Input: part model. Units: mm. Frame: model coordinates. A direction names the side the tool comes from. Round coordinates to 2 decimals unless told otherwise and drop trailing zeros. Write each loop counter-clockwise with the first axis right and the second up, starting at its lowest first coordinate (ties: lowest second). Pieces come first, ordered by that corner, then holes. Notation, with made-up numbers: (22, 20.25) - (47, 20.25) arc R25 ccw to (47, 33.25) - close; hole circle Ø8 at (60.25, 83). An arc over 180 degrees is marked (long way). Use one line per item in the form item = value.
```python
from build123d import *

# Parameters (mm, degrees)
SKETCH1_W           = 40
SKETCH1_H           = 40
SKETCH1_R           = 1.5
SKETCH1_R_2         = 2.8
BOSS_EXTRUDE1_DEPTH = 5.7
BOSS_EXTRUDE3_START = 5.7
SKETCH1_3_W         = 40
SKETCH1_3_H         = 40
SKETCH1_3_R         = 2.8
SKETCH1_3_R_2       = 1.5
BOSS_EXTRUDE3_DEPTH = 3.4
SKETCH4_W           = 3.5
SKETCH4_H           = 40
CUT_EXTRUDE2_DEPTH  = 4
SKETCH2_W           = 3
SKETCH2_H           = 40
BOSS_EXTRUDE4_DEPTH = 5.1
CUT_EXTRUDE3_START  = -39.5
SKETCH5_R           = 2
CUT_EXTRUDE3_DEPTH  = 33
CUT_EXTRUDE4_START  = -5.1
SKETCH6_W           = 3.85
SKETCH6_H           = 5.76
CUT_EXTRUDE4_DEPTH  = 5.1
FILLET1_R           = 0.62
CHAMFER1_SIZE       = 1.4
CHAMFER1_SIZE2      = 3.144451483


with BuildPart() as part:
    # Sketch1 → Boss-Extrude1 (new body)
    # profile 1 of 7: a face of its own
    with BuildSketch(Plane(origin=(0, 0, 0), x_dir=(1, 0, 0), z_dir=(0, 1, 0))):
        Rectangle(SKETCH1_W, SKETCH1_H)
        with Locations((0, -10)):
            Circle(SKETCH1_R, mode=Mode.SUBTRACT)
        with Locations((0, 10)):
            Circle(SKETCH1_R, mode=Mode.SUBTRACT)
        with Locations(Location((-16.2, -10, 0), (0, 0, 270))):
            Circle(SKETCH1_R, mode=Mode.SUBTRACT)
        with Locations(Location((16.2, -10, 0), (0, 0, 270))):
            Circle(SKETCH1_R, mode=Mode.SUBTRACT)
        with Locations(Location((16.2, 10, 0), (0, 0, 270))):
            Circle(SKETCH1_R, mode=Mode.SUBTRACT)
        with Locations(Location((-16.2, 10, 0), (0, 0, 270))):
            Circle(SKETCH1_R, mode=Mode.SUBTRACT)
    # profile 2 of 7: a face of its own
    with BuildSketch(Plane(origin=(0, 0, 0), x_dir=(1, 0, 0), z_dir=(0, 1, 0))):
        with Locations((0, 10)):
            Circle(SKETCH1_R)
    # profile 3 of 7: a face of its own
    with BuildSketch(Plane(origin=(0, 0, 0), x_dir=(1, 0, 0), z_dir=(0, 1, 0))):
        with Locations((0, -10)):
            Circle(SKETCH1_R)
    # profile 4 of 7: a face of its own
    with BuildSketch(Plane(origin=(0, 0, 0), x_dir=(1, 0, 0), z_dir=(0, 1, 0))):
        with Locations((-16.2, 10)):
            Circle(SKETCH1_R_2)
        with Locations(Location((-16.2, 10, 0), (0, 0, 270))):
            Circle(SKETCH1_R, mode=Mode.SUBTRACT)
    # profile 5 of 7: a face of its own
    with BuildSketch(Plane(origin=(0, 0, 0), x_dir=(1, 0, 0), z_dir=(0, 1, 0))):
        with Locations((-16.2, -10)):
            Circle(SKETCH1_R_2)
        with Locations(Location((-16.2, -10, 0), (0, 0, 270))):
            Circle(SKETCH1_R, mode=Mode.SUBTRACT)
    # profile 6 of 7: a face of its own
    with BuildSketch(Plane(origin=(0, 0, 0), x_dir=(1, 0, 0), z_dir=(0, 1, 0))):
        with Locations((16.2, 10)):
            Circle(SKETCH1_R_2)
        with Locations(Location((16.2, 10, 0), (0, 0, 270))):
            Circle(SKETCH1_R, mode=Mode.SUBTRACT)
    # profile 7 of 7: a face of its own
    with BuildSketch(Plane(origin=(0, 0, 0), x_dir=(1, 0, 0), z_dir=(0, 1, 0))):
        with Locations((16.2, -10)):
            Circle(SKETCH1_R_2)
        with Locations(Location((16.2, -10, 0), (0, 0, 270))):
            Circle(SKETCH1_R, mode=Mode.SUBTRACT)
    extrude(amount=BOSS_EXTRUDE1_DEPTH)

    # Sketch1_3 → Boss-Extrude3 (add)
    # profile 1 of 3: a face of its own
    with BuildSketch(Plane(origin=(0, 0, 0), x_dir=(1, 0, 0), z_dir=(0, 1, 0)).offset(BOSS_EXTRUDE3_START)):
        Rectangle(SKETCH1_3_W, SKETCH1_3_H)
        with Locations(Location((16.2, 10, 0), (0, 0, 270))):
            Circle(SKETCH1_3_R, mode=Mode.SUBTRACT)
        with Locations(Location((-16.2, 10, 0), (0, 0, 270))):
            Circle(SKETCH1_3_R, mode=Mode.SUBTRACT)
        with Locations((0, -10)):
            Circle(SKETCH1_3_R_2, mode=Mode.SUBTRACT)
        with Locations((0, 10)):
            Circle(SKETCH1_3_R_2, mode=Mode.SUBTRACT)
        with Locations(Location((-16.2, -10, 0), (0, 0, 270))):
            Circle(SKETCH1_3_R, mode=Mode.SUBTRACT)
        with Locations(Location((16.2, -10, 0), (0, 0, 270))):
            Circle(SKETCH1_3_R, mode=Mode.SUBTRACT)
    # profile 2 of 3: a face of its own
    with BuildSketch(Plane(origin=(0, 0, 0), x_dir=(1, 0, 0), z_dir=(0, 1, 0)).offset(BOSS_EXTRUDE3_START)):
        with Locations((0, 10)):
            Circle(SKETCH1_3_R_2)
    # profile 3 of 3: a face of its own
    with BuildSketch(Plane(origin=(0, 0, 0), x_dir=(1, 0, 0), z_dir=(0, 1, 0)).offset(BOSS_EXTRUDE3_START)):
        with Locations((0, -10)):
            Circle(SKETCH1_3_R_2)
    extrude(amount=BOSS_EXTRUDE3_DEPTH)

    # Sketch4 → Cut-Extrude2 (cut)
    with BuildSketch(Plane.XZ):
        with Locations((18.25, 0)):
            Rectangle(SKETCH4_W, SKETCH4_H)
        with Locations((-18.25, 0)):
            Rectangle(SKETCH4_W, SKETCH4_H)
    extrude(amount=-CUT_EXTRUDE2_DEPTH, mode=Mode.SUBTRACT)

    # Sketch2 → Boss-Extrude4 (add)
    with BuildSketch(Plane(origin=(0, 9.1, 0), x_dir=(1, 0, 0), z_dir=(0, 1, 0))):
        with Locations((-21.5, 0)):
            Rectangle(SKETCH2_W, SKETCH2_H)
        with Locations((21.5, 0)):
            Rectangle(SKETCH2_W, SKETCH2_H)
    extrude(amount=-BOSS_EXTRUDE4_DEPTH)

    # Sketch5 → Cut-Extrude3 (cut)
    with BuildSketch(Plane(origin=(23, 0, 0), x_dir=(0, 0, -1), z_dir=(1, 0, 0)).offset(CUT_EXTRUDE3_START)):
        with Locations((16, 0)):
            Circle(SKETCH5_R)
        with Locations((-16, 0)):
            Circle(SKETCH5_R)
    extrude(amount=CUT_EXTRUDE3_DEPTH, mode=Mode.SUBTRACT)

    # Sketch6 → Cut-Extrude4 (cut)
    with BuildSketch(Plane(origin=(0, 9.1, 0), x_dir=(1, 0, 0), z_dir=(0, 1, 0)).offset(CUT_EXTRUDE4_START)):
        with Locations((21.075, 3.36)):
            Rectangle(SKETCH6_W, SKETCH6_H)
    extrude(amount=CUT_EXTRUDE4_DEPTH, mode=Mode.SUBTRACT)

    # Fillet1
    fillet1_edges = [part.edges().sort_by_distance(p)[0] for p in [
        (19.15, 6.55, -0.48),
        (19.15, 6.55, -6.24),
    ]]
    fillet(fillet1_edges, radius=FILLET1_R)

    # Chamfer1
    chamfer1_edges = [part.edges().sort_by_distance(p)[0] for p in [
        (-23, 9.1, 0),
    ]]
    chamfer1_side = [part.faces().sort_by_distance(p)[0] for p in [
        (-0.269953671, 9.1, 0.043011548),
    ]]
    chamfer(chamfer1_edges, length=CHAMFER1_SIZE, length2=CHAMFER1_SIZE2, reference=chamfer1_side[0])


solid = part.part
```
(1) Access query for faces 4 (the face through (16.5, 2.4, -15.8)), 5 (the face through (21, 7, -6.24)), 6 (the face through (-16.5, 2.4, 15.7)), 7 (the face through (18.56, 7.38, -8.49)). Directions: +Z, -Z, +X, -X, +Y, -Y. A direction counts if a zero-diameter tool reaches every point of the face in a straight line with its end or side. Return the directions, or none.
Derived:
face_4 = +Z, -Z, +X, -Y
face_5 = +X, +Y, -Y
face_6 = +Z, -Z, -X, -Y
face_7 = +Y
(2) Cut plane C-C on x = -2. Output: boundary loops of the cut face in (y, z).
Derived:
outline = (0, -20) - (9.1, -20) - (9.1, 20) - (0, 20) - (0, 18) arc R2 cw to (0, 14) - (0, -14) arc R2 cw to (0, -18) - close
(3) Material intervals for L1, parallel to Z at x = -16.2, y = 3.15; L2, parallel to Z at x = -16.2, y = 1.2; L3, parallel to Z at x = 17.5, y = 8.25, sorted ascending.
Derived:
L1 = -20 to -11.5, -8.5 to 8.5, 11.5 to 20
L2 = -20 to -17.6, -14.4 to -11.5, -8.5 to 8.5, 11.5 to 14.4, 17.6 to 20
L3 = -20 to -12.48, -7.52 to 7.52, 12.48 to 20
(4) First-contact query: pin 1 Ø2 at (y, z) = (2, -16) entering from +X; pin 2 Ø1.7 at (x, z) = (-17, 8.5) entering from +Y; pin 3 Ø5 at (x, z) = (20, 2.5) entering from -Y. Flat tips, straight axial feed; report the tip coordinate or a pass-through.
Derived:
pin_1 = 16.5
pin_2 = 5.7
pin_3 = 4
(5) Draft query along X for faces 1 (the face through (16.5, 2.4, 15.7)), 2 (the face through (-14.713, 3.443, -10.195)), 3 (the face through (0, 0, 19)). Return one class per face: released by +X, released by -X, zero draft, split by the parting line, or undercut.
Derived:
face_1 = released by +X
face_2 = undercut
face_3 = zero draft
(6) Cut plane B-B on y = 2.75. Output: boundary loops of the cut face in (x, z), then the cut area to 3 significant figures.
Derived:
outline = (-16.5, -20) - (16.5, -20) - (16.5, -11.47) arc R1.5 cw (long way) to (16.5, -8.53) - (16.5, 8.53) arc R1.5 cw (long way) to (16.5, 11.47) - (16.5, 20) - (-16.5, 20) - (-16.5, 11.47) arc R1.5 cw (long way) to (-16.5, 8.53) - (-16.5, -8.53) arc R1.5 cw (long way) to (-16.5, -11.47) - close
area = 1,300 mm^2
(7) Cut plane D-D on z = 16. Output: boundary loops of the cut face in (x, y), then the cut area to 3 significant figures.
Derived:
outline = (-23, 4) - (-16.5, 4) - (-16.5, 2) - (16.5, 2) - (16.5, 4) - (23, 4) - (23, 9.1) - (-21.6, 9.1) - (-23, 5.96) - close
area = 298 mm^2
(8) Cut plane A-A on z = -10. Output: boundary loops of the cut face in (x, y).
Derived:
outline = (-23, 4) - (-17.7, 4) - (-17.7, 5.7) - (-19, 5.7) - (-19, 9.1) - (-21.6, 9.1) - (-23, 5.96) - close; (-14.7, 0) - (14.7, 0) - (14.7, 5.7) - (13.4, 5.7) - (13.4, 9.1) - (-13.4, 9.1) - (-13.4, 5.7) - (-14.7, 5.7) - close; (17.7, 4) - (23, 4) - (23, 9.1) - (19, 9.1) - (19, 5.7) - (17.7, 5.7) - close
